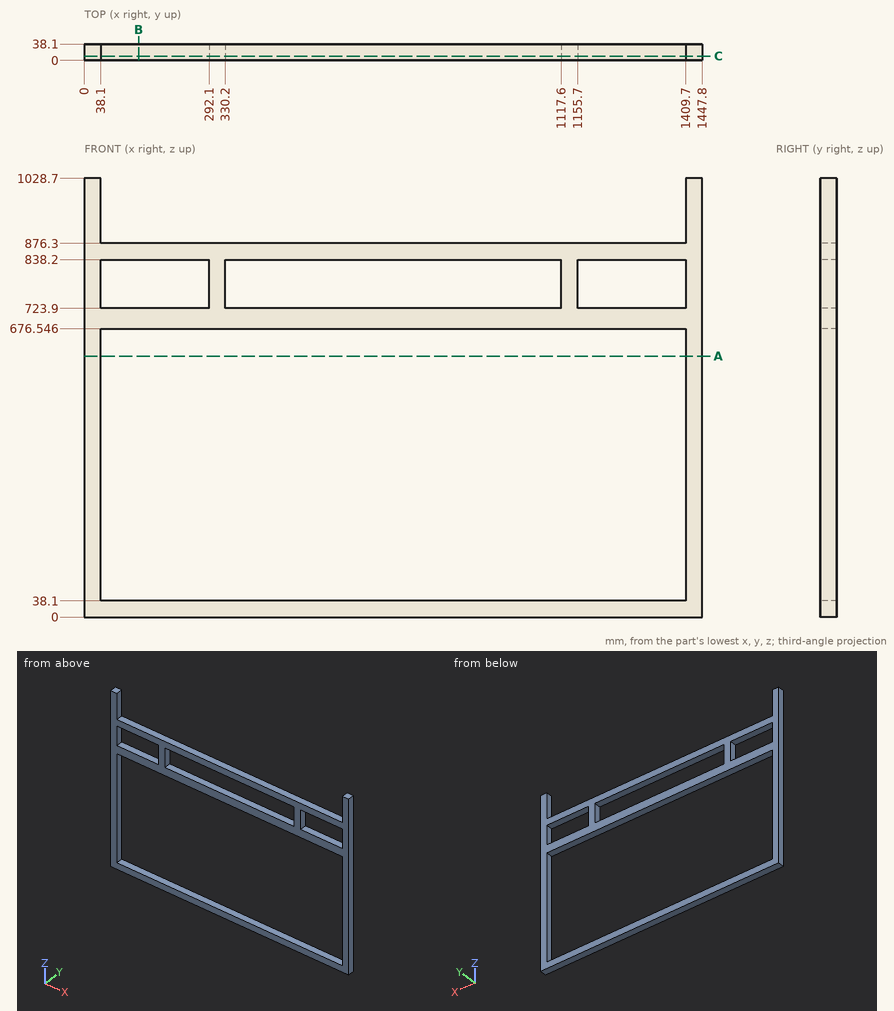
Job drawing, mm, ordinate dimensions from the low corner. One solid piece. Round coordinates to 2 decimals unless told otherwise and drop trailing zeros. Loops run counter-clockwise (first coordinate to the right, second up) from the corner with the lowest first, then second, coordinate; pieces in that order, holes last.
(1) Drop a flat-ended pin along its axis: pin 1 (19 mm diameter, centred on x = 1305, y = 15.5, fed in from +Z). Give the stop position or say it passes through.
(2) Cut at C-C (y = 9.5). Give the cut face in (x, z), plus the area to 3 significant figures.
(3) Wall check: line 1 along Z through (x, y) = (244, 31); line 2 along X through (y, z) = (34, 763.5); line 3 along X through (y, z) = (11, 291). Give the ranges that are in metal, low to high.
(4) Cut at B-B (x = 127). Give the cut face in (y, z), plus the area to 3 significant figures.
(5) Cut at A-A (z = 612). Give the cut face in (x, y), plus the area to 3 significant figures.
Findings below:
1. pin 1: stops at z = 876.3
2. outline: (0, 0) - (1447.8, 0) - (1447.8, 1028.7) - (1409.7, 1028.7) - (1409.7, 876.3) - (38.1, 876.3) - (38.1, 1028.7) - (0, 1028.7) - close; hole (38.1, 38.1) - (1409.7, 38.1) - (1409.7, 676.55) - (38.1, 676.55) - close; hole (38.1, 723.9) - (292.1, 723.9) - (292.1, 838.2) - (38.1, 838.2) - close; hole (330.2, 723.9) - (1117.6, 723.9) - (1117.6, 838.2) - (330.2, 838.2) - close; hole (1155.7, 723.9) - (1409.7, 723.9) - (1409.7, 838.2) - (1155.7, 838.2) - close
2. area: 257,000 mm2
3. line 1: z = 0 to 38.1, 676.55 to 723.9, 838.2 to 876.3
3. line 2: x = 0 to 38.1, 292.1 to 330.2, 1117.6 to 1155.7, 1409.7 to 1447.8
3. line 3: x = 0 to 38.1, 1409.7 to 1447.8
4. outline: (0, 0) - (38.1, 0) - (38.1, 38.1) - (0, 38.1) - close; (0, 676.55) - (38.1, 676.55) - (38.1, 723.9) - (0, 723.9) - close; (0, 838.2) - (38.1, 838.2) - (38.1, 876.3) - (0, 876.3) - close
4. area: 4,710 mm2
5. outline: (0, 0) - (38.1, 0) - (38.1, 38.1) - (0, 38.1) - close; (1409.7, 0) - (1447.8, 0) - (1447.8, 38.1) - (1409.7, 38.1) - close
5. area: 2,900 mm2
